Part print with two shaded views. Sizes in mm from the minimum x, y, z corner. Coordinates: 2 decimals unless noted, no trailing zeros. Order: outer loops, then holes, each group sorted by start corner. A loop starts at its lowest first (then second) coordinate and runs counter-clockwise, first axis right, second up. Notation, with made-up numbers: (23, -17.75) - (76, -17.75) arc R30 ccw to (76, 18.25) - close; hole circle Ø10 at (7, 66.25). An arc over 180 degrees is marked (long way). One line per item, written item: value.
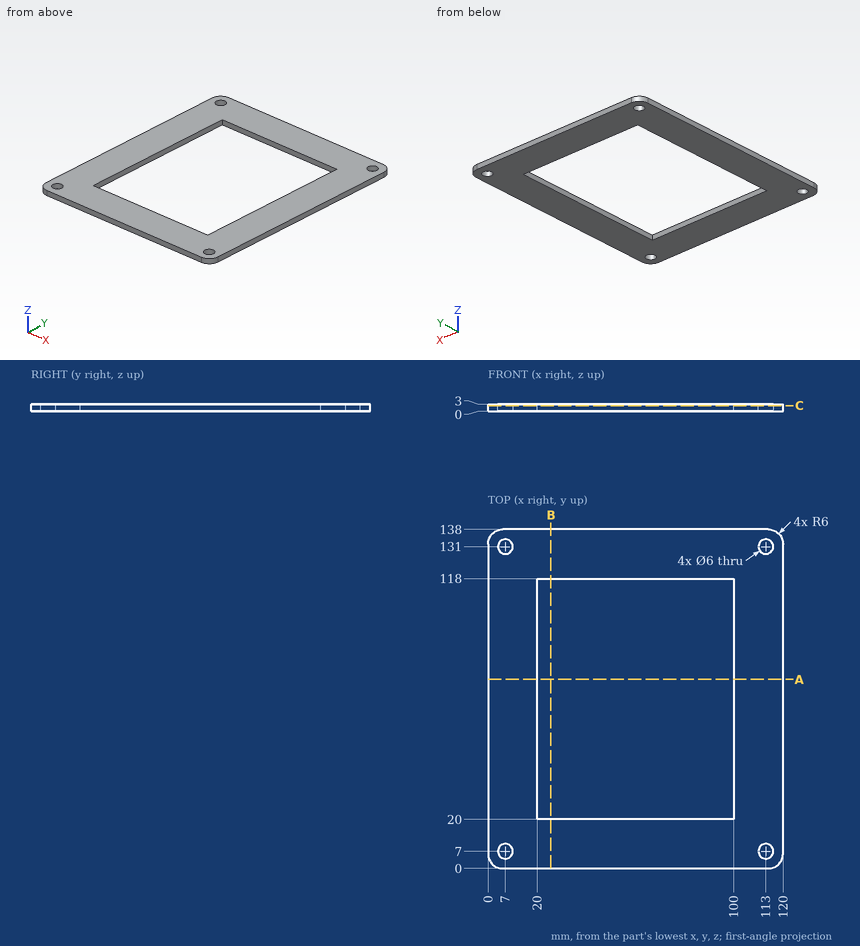
1. Band-saw the part on A-A, the plane y = 77. Give the cut face in (x, z), and give its area (3 significant figures).
Values found:
outline: (0, 0) - (20, 0) - (20, 3) - (0, 3) - close; (100, 0) - (120, 0) - (120, 3) - (100, 3) - close
area: 120 mm2
2. Band-saw the part on B-B, the plane x = 25.5. Give the cut face in (y, z), and give its area (3 significant figures).
Values found:
outline: (0, 0) - (20, 0) - (20, 3) - (0, 3) - close; (118, 0) - (138, 0) - (138, 3) - (118, 3) - close
area: 120 mm2
3. Band-saw the part on C-C, the plane z = 2.3. Give the cut face in (x, y), and give its area (3 significant figures).
Values found:
outline: (0, 6) arc R6 ccw to (6, 0) - (114, 0) arc R6 ccw to (120, 6) - (120, 132) arc R6 ccw to (114, 138) - (6, 138) arc R6 ccw to (0, 132) - close; hole circle Ø6 at (7, 7); hole circle Ø6 at (7, 131); hole (20, 20) - (100, 20) - (100, 118) - (20, 118) - close; hole circle Ø6 at (113, 7); hole circle Ø6 at (113, 131)
area: 8,580 mm2
4. Probe line 1 along Y through (x, z) = (7, 1.4); line 2 along X through (y, z) = (52.5, 2.4); line 3 along Y through (x, z) = (90, 1.9). List the from-to ranges inside material, lowest first.
Values found:
line 1: y = 0 to 4, 10 to 128, 134 to 138
line 2: x = 0 to 20, 100 to 120
line 3: y = 0 to 20, 118 to 138
